Geometry check sheet. Reference: the model listing, model coordinates, mm. A direction names the side the tool comes from. Coordinates: 2 decimals unless noted, no trailing zeros. Order: outer loops, then holes, each group sorted by start corner. A loop starts at its lowest first (then second) coordinate and runs counter-clockwise, first axis right, second up.
```python
from build123d import *

# Parameters (mm, degrees)
CROQUIS1_R              = 7.9375
SALIENTE_EXTRUIR1_DEPTH = 20
CROQUIS2_R              = 15
SALIENTE_EXTRUIR2_DEPTH = 50
REDONDEO1_R             = 10
CROQUIS3_W              = 5
CROQUIS3_H              = 21.165863944
CORTAR_EXTRUIR1_DEPTH   = 16
CROQUIS4_R              = 3
CORTAR_EXTRUIR2_DEPTH   = 10
CROQUIS5_W              = 4
CROQUIS5_H              = 2
CORTAR_EXTRUIR3_DEPTH   = 39


with BuildPart() as part:
    # Croquis1 → Saliente-Extruir1 (new body)
    with BuildSketch(Plane.XY):
        Circle(CROQUIS1_R)
    extrude(amount=-SALIENTE_EXTRUIR1_DEPTH)

    # Croquis2 → Saliente-Extruir2 (add)
    with BuildSketch(Plane(origin=(0, 0, -20), x_dir=(-1, 0, 0), z_dir=(0, 0, -1))):
        Circle(CROQUIS2_R)
    extrude(amount=SALIENTE_EXTRUIR2_DEPTH)

    # Redondeo1
    # the kernel refuses this fillet: 10 mm, written as the material it takes off along each edge
    with BuildSketch(Plane(origin=(0, 0, -20), x_dir=(-1, 0, 0), z_dir=(0, -1, 0))) as redondeo1_piece_1:
        with BuildLine():
            CenterArc((5, 9.558822822), REDONDEO1_R, 287.082597034, 72.917402966)
            Line((7.9375, 0), (7.99625, -0.191176456))
            ThreePointArc((7.99625, -0.191176456), (11.46875, -0.2), (15, -0.2))
            Line((15, -0.2), (15.2, 0))
            Line((15.2, 0), (15.2, 9.558822822))
            Line((15.2, 9.558822822), (15, 9.558822822))
        make_face()
    revolve(axis=Axis((0, 0, -20), (0, 0, -1)), mode=Mode.SUBTRACT)

    # Croquis3 → Cortar-Extruir1 (cut)
    with BuildSketch(Plane.XY):
        Rectangle(CROQUIS3_W, CROQUIS3_H)
    extrude(amount=-CORTAR_EXTRUIR1_DEPTH, mode=Mode.SUBTRACT)

    # Croquis4 → Cortar-Extruir2 (cut, symmetric)
    with BuildSketch(Plane(origin=(0, 0, 0), x_dir=(0, 0, -1), z_dir=(1, 0, 0))):
        with Locations((5, 0)):
            Circle(CROQUIS4_R)
    extrude(amount=CORTAR_EXTRUIR2_DEPTH, both=True, mode=Mode.SUBTRACT)

    # Croquis5 → Cortar-Extruir3 (cut)
    with BuildSketch(Plane(origin=(0, 0, -70), x_dir=(-1, 0, 0), z_dir=(0, 0, -1))):
        with Locations((0, 15)):
            Rectangle(CROQUIS5_W, CROQUIS5_H)
        with Locations((0, -15)):
            Rectangle(CROQUIS5_W, CROQUIS5_H)
    extrude(amount=-CORTAR_EXTRUIR3_DEPTH, mode=Mode.SUBTRACT)


solid = part.part
```
Item 1: Depth check by flat-ended pin: P1, Ø12, axis at y = 1, z = -7.5, coming from the -X side; P2, Ø3, axis at x = 1.5, y = 5, coming from the +Z side; P3, Ø6, axis at y = -11, z = -23, coming from the +X side; P4, Ø1.5, axis at x = -11, y = -8.5, coming from the +Z side. Enter the tip coordinate at first touch or a pass-through.
Item 2: Thickness scan on line 1 along Z through (x, y) = (-6, 0); line 2 along Y through (x, z) = (-5, -5); line 3 along Z through (x, y) = (0.5, 0). Record the ranges inside material, lowest first.
Item 3: Sectioned sample at C-C (y = 0). Give the number of separate pieces and of enclosed holes in the cut face, and give its area (3 significant figures).
Item 4: Tool access check on faces 5 (the face through (7.332, -3.04, -9.86)), 6 (the face through (0, -14, -51)), 7 (the face through (0, 14, -51)), 8 (the face through (2.5, 0, -10)), 9 (the face through (0, 0, -70)). Record the directions out of +Z, -Z, +X, -X, +Y, -Y that give a thin tool (end or side, any length) a straight path to the whole face; none if there is none.
Item 5: Sectioned sample at A-A (z = -39). Record the cut outline in (x, y).
Item 6: Release check for a two-part mould opening along Z. For faces 1 (the face through (-2.5, 0, -10)), 2 (the face through (-5, 0, -2)), 3 (the face through (5, 0, -2)), 4 (the face through (0, 0, -16)) record: pulls with the +Z half, pulls with the -Z half, needs draft (parallel to the pull), parting line crosses it, or undercut.
Item 7: Sectioned sample at B-B (z = -5). Record the cut outline in (x, y) (1 decimal), and give its area (3 significant figures).
Item 8: Sectioned sample at D-D (z = -18.5). Record the cut outline in (x, y) (1 decimal), and give its area (3 significant figures).
Geometry check:
1. P1: stops at x = -7.94
1. P2: stops at z = 0
1. P3: stops at x = 10.79
1. P4: stops at z = -23.77
2. line 1: z = -70 to -8, -2 to 0
2. line 2: y = -6.16 to -3, 3 to 6.16
2. line 3: z = -70 to -16
3. separate pieces: 3
3. enclosed holes: 0
3. area: 1,640 mm2
4. face 5: +Z
4. face 6: -Z, -Y
4. face 7: -Z, +Y
4. face 8: +Z, +Y, -Y
4. face 9: -Z, +X, -X, +Y, -Y
5. outline: (-2, -14.87) - (-2, -14) - (2, -14) - (2, -14.87) arc R15 ccw to (2, 14.87) - (2, 14) - (-2, 14) - (-2, 14.87) arc R15 ccw to start
6. face 1: needs draft
6. face 2: undercut
6. face 3: undercut
6. face 4: pulls with the +Z half
7. outline: (-7.3, -3) arc R7.9 ccw to (-2.5, -7.5) - (-2.5, -3) - close; (-7.3, 3) - (-2.5, 3) - (-2.5, 7.5) arc R7.9 ccw to start; (2.5, -7.5) arc R7.9 ccw to (7.3, -3) - (2.5, -3) - close; (2.5, 3) - (7.3, 3) arc R7.9 ccw to (2.5, 7.5) - close
7. area: 57.0 mm2
8. outline: circle Ø15.9 at (0, 0)
8. area: 198 mm2
